Input: dimensioned drawing with shaded views. Units: mm. Origin: part minimum x, y, z. A direction names the side the tool comes from. Give positions to 0.01 mm unless a question says otherwise; leave off trailing zeros. Loops run counter-clockwise (first coordinate to the right, second up) from the corner with the lowest first, then second, coordinate; pieces in that order, holes last.
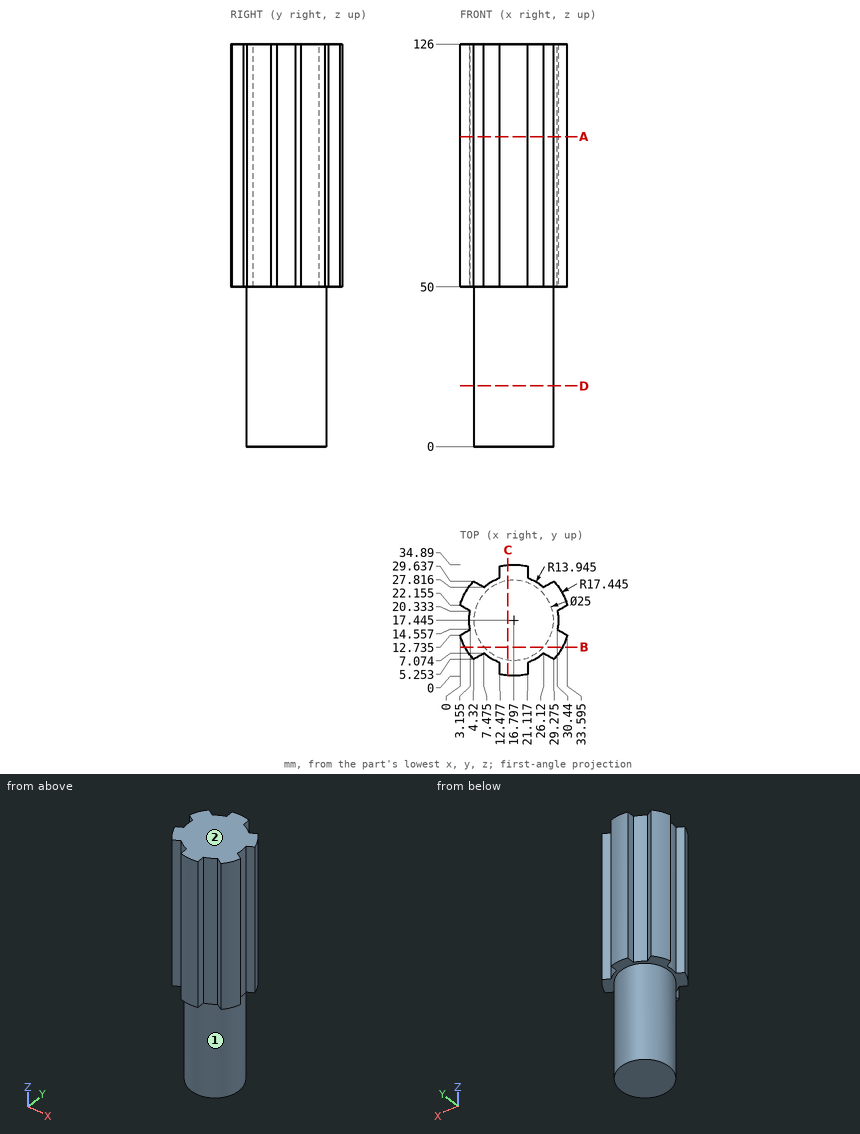
Item 1: Set-up query: the marked faces 1 and 2. Return all of +Z, -Z, +X, -X, +Y, -Y with unobstructed straight access to the full face (end or side cutting, diameter ignored); none if empty.
Values follow:
face 1: -Z
face 2: +Z, +X, -X, +Y, -Y
Item 2: Pin query (flat end, axial travel): pin 1 (10 mm diameter, centred on x = 25.5, z = 74, fed in from +Y); pin 2 (2 mm diameter, centred on y = 17.5, z = 104.5, fed in from +X); pin 3 (1.8 mm diameter, centred on y = 2, z = 76, fed in from +X). Return the tip coordinate at first contact, or that it passes through.
Values follow:
pin 1: stops at y = 34.49
pin 2: stops at x = 30.74
pin 3: stops at x = 21.12
Item 3: Section query C-C on x = 15. Return loops of the section in (y, z) (1 decimal), plus the area to 3 significant figures.
Values follow:
outline: (0.1, 50) - (5.1, 50) - (5.1, 0) - (29.8, 0) - (29.8, 50) - (34.8, 50) - (34.8, 126) - (0.1, 126) - close
area: 3,870 mm2
Item 4: Ray query, probe 1 along Z at (x, y) = (2, 9.5); probe 2 along X at (y, z) = (33, 76.5); probe 3 along Y at (x, z) = (17, 70.5). Return the intervals inside material, ascending.
Values follow:
probe 1: z = 50 to 126
probe 2: x = 12.48 to 21.12
probe 3: y = 0 to 34.89
Item 5: Section query D-D on z = 19. Return loops of the section in (x, y) (1 decimal).
Values follow:
outline: circle Ø25 at (16.8, 17.4)
Item 6: Section query B-B on y = 9. Return loops of the section in (x, z), plus the area to 3 significant figures.
Values follow:
outline: (1.53, 50) - (7.58, 50) - (7.58, 0) - (26.01, 0) - (26.01, 50) - (32.06, 50) - (32.06, 126) - (1.53, 126) - close
area: 3,240 mm2
Item 7: Section query A-A on z = 97. Return loops of the section in (x, y) (1 decimal).
Values follow:
outline: (0, 12.7) arc R17.4 ccw to (4.3, 5.3) - (7.5, 7.1) arc R13.9 ccw to (12.5, 4.2) - (12.5, 0.5) arc R17.4 ccw to (21.1, 0.5) - (21.1, 4.2) arc R13.9 ccw to (26.1, 7.1) - (29.3, 5.3) arc R17.4 ccw to (33.6, 12.7) - (30.4, 14.6) arc R13.9 ccw to (30.4, 20.3) - (33.6, 22.2) arc R17.4 ccw to (29.3, 29.6) - (26.1, 27.8) arc R13.9 ccw to (21.1, 30.7) - (21.1, 34.3) arc R17.4 ccw to (12.5, 34.3) - (12.5, 30.7) arc R13.9 ccw to (7.5, 27.8) - (4.3, 29.6) arc R17.4 ccw to (0, 22.2) - (3.2, 20.3) arc R13.9 ccw to (3.2, 14.6) - close
